Here's how the part is built. I have some questions about the finished solid (model axes, mm). A direction names the side the tool comes from. Round coordinates to 2 decimals unless told otherwise and drop trailing zeros. Order: outer loops, then holes, each group sorted by start corner. A loop starts at its lowest first (then second) coordinate and runs counter-clockwise, first axis right, second up. Notation, with made-up numbers: (55, -34) -> (90, -34) arc R18 ccw to (90, -30) -> close; hole circle Ø1 at (0.25, 68). An arc over 180 degrees is marked (long way). Use a Markdown table: item, result. Add a question column.
(1) I want a section at B-B, the plane z = -1. Please give me the cut outline in (x, y), then the cut area to 3 significant figures.
(2) I want a section at C-C, the plane x = 4. Give the number of separate pieces and of enclosed holes in the cut face, then the cut area to 3 significant figures.
(3) I want a section at A-A, the plane x = 0. Please give me the cut outline in (y, z), then the cut area to 3 significant figures.
(4) I'm going to push flat-ended pins straight in: P1, Ø10, axis at x = 2, z = -15.5, coming from the +Y side; P2, Ø4, axis at x = 12, y = 45.5, coming from the +Z side; P3, Ø5, axis at x = 4.5, y = 31, coming from the -Z side; P4, Ø10, axis at x = 2.5, z = -0.5, coming from the -Y side. Where does each tip first touch, or does it pass through?
(5) Thinking about a two-plate mould opening in Y: for faces 1 (the face through (-18.369, 29, 0)), 2 (the face through (-17.45, 36.35, -3.61)), 3 (the face through (0.861, 62.494, -16.123)), which applies, pulls with the +Y half, pulls with the -Y half, needs draft (parallel to the pull), parting line crosses it, or undercut?
(6) On a 3-axis mill with a long thin cutter (end or side, diameter ignored), from which of +Z, -Z, +X, -X, +Y, -Y can I reach the whole of each face in a straight line? I mean faces 4 (the face through (0, 28, 0)), 5 (the face through (1, 58, -21.7)), 6 (the face through (4.5, 58, -18)). Say none if no direction works.
(7) If I drill on probe 1 along X at (y, z) = (45, -7.5); probe 2 along Y at (x, z) = (0, -12.25); probe 3 along Y at (x, z) = (0, -9.25), over which ranges is the centre line in solid material (lowest first)?
(8) I want a section at D-D, the plane z = -8. Please give me the cut outline in (x, y), then the cut area to 3 significant figures.
Autodesk Inventor part; units mm, degrees
ref_plane "Work Plane2" through (0, 61, 0) normal (0, 1, 0) x (-1, 0, 0)
ref_plane "YZ Plane" through (0, 0, 0) normal (1, 0, 0) x (0, 1, 0)
ref_plane "XY Plane" through (0, 0, 0) normal (0, 0, 1) x (1, 0, 0)
sketch "Sketch1" plane through (0, 0, 0) normal (0, 0, 1) x (1, 0, 0)
  circle A0 centre (0, 0) radius 11
  line L0 (-9.5, 5.5453) -> (-9.5, -5.5453)
  line L1 (9.5, 5.5453) -> (9.5, -5.5453)
  circle A1 centre (0, 0) radius 32.5
  dimension "d0" = 22
  dimension "d1" = 19
  dimension "d2" = 65
extrude "Extrusion1" add sketch "Sketch1" along normal blind 3.3 contours A0 L1 | L0 A0 | A1
sketch "Sketch2" plane through (0, 0, 0) normal (1, 0, 0) x (0, 1, 0)
  line L0 (32.5, 0) -> (-32.5, 0)
  line L1 (32.5, 0) -> (55.5, -21.7)
  line L2 (55.5, -21.7) -> (62.5, -21.7)
  line L3 (62.5, -21.7) -> (62.5, -10.7)
  line L4 (32.5, 3.3) -> (-32.5, 3.3)
  line L5 (32.5, 3.3) -> (62.5, -10.7)
  line L6 (0, 0) -> (0, -19.375) construction
  line L7 (32.5, 3.3) -> (32.5, 0)
  dimension "d8" = 7
  dimension "d9" = 25
  dimension "d10" = 11
  dimension "d11" = 30
revolve "Revolution1" add sketch "Sketch2" angle 360 about axis through (0, 0, 0) along (0, 0, -1)
fillet "Fillet1" radius 10 1 edges at (0, -32.5, 3.3)
ref_plane "Work Plane2" through (0, 61, 0) normal (0, 1, 0) x (-1, 0, 0)
sketch "Sketch3" plane through (0, 61, 0) normal (0, 1, 0) x (-1, 0, 0)
  circle A0 centre (0, -16.2) radius 4.5
  line L0 (4.5, -16.2) -> (4.5, -20.7)
  line L1 (-4.5, -20.7) -> (-4.5, -16.2)
  line L2 (-62.5, -21.7) -> (62.5, -21.7)
  line L3 (62.5, -21.7) -> (62.5, -11.7) construction
  line L4 (62.5, -10.7) -> (62.5, -21.7)
  line L5 (-9.5, 0) -> (9.5, 0)
  line L6 (-4.5, -20.7) -> (4.5, -20.7)
  point P0 (0, 0)
  point P1 (0, 0)
  point P2 (0, -20.7)
  dimension "d14" = 9
  dimension "d22" = 1
extrude "Extrusion2" cut sketch "Sketch3" against normal blind 6
sketch "Sketch4" plane through (0, 0, 3.3) normal (0, 0, 1) x (1, 0, 0)
  circle A0 centre (0, 45) radius 9
  point P0 (0, 0)
  dimension "d25" = 45
  dimension "d26" = 18
extrude "Extrusion3" cut sketch "Sketch4" against normal through all
pattern_circular "Circular Pattern1" count 10 over 360 about axis through (0, 0, -6.7) along (0, 0, 1) of "Extrusion3"
sketch "Sketch5" plane through (0, 0, -21.7) normal (0, 0, -1) x (-1, 0, 0)
  line L0 (82.923, -74.4217) -> (-85.9985, -74.4217)
  line L1 (-85.9985, -74.4217) -> (-85.9985, 73.4258)
  line L2 (-85.9985, 73.4258) -> (82.923, 73.4258)
  line L3 (82.923, 73.4258) -> (82.923, -74.4217)
  line L4 (-19.4974, 63.9822) -> (18.3694, 63.9822)
  line L5 (18.3694, 63.9822) -> (18.3694, 24.2787)
  line L6 (18.3694, 24.2787) -> (-19.4974, 24.2787)
  line L7 (-19.4974, 24.2787) -> (-19.4974, 63.9822)
  point P0 (0, 0)
extrude "Extrusion4" cut sketch "Sketch5" against normal through all
properties part number "CVT_Ring"
Taken from the geometry:
| question | item | result |
|---|---|---|
| 1 | outline | (-18.37, 28.09) arc R33.56 cw to (19.5, 27.32) -> (19.5, 30.69) arc R9 cw to (17.56, 37.84) arc R41.71 ccw to (8.03, 40.93) arc R9 cw to (-8.03, 40.93) arc R41.71 ccw to (-17.56, 37.84) arc R9 cw to (-18.37, 32.44) -> close |
| 1 | area | 245 mm2 |
| 2 | separate pieces | 2 |
| 2 | enclosed holes | 1 |
| 2 | area | 127 mm2 |
| 3 | outline | (24.28, 0) -> (32.5, 0) -> (36, -3.3) -> (36, 1.67) -> (34.51, 2.36) arc R10 ccw to (30.28, 3.3) -> (24.28, 3.3) -> close; (54, -20.28) -> (55.5, -21.7) -> (62.5, -21.7) -> (62.5, -10.7) -> (54, -6.73) -> close; hole (55, -20.7) -> (61, -20.7) -> (61, -11.7) -> (55, -11.7) -> close |
| 3 | area | 96.5 mm2 |
| 4 | P1 | stops at y = 62.5 |
| 4 | P2 | stops at z = -2.56 |
| 4 | P3 | stops at z = -1.25 |
| 4 | P4 | stops at y = 24.28 |
| 5 | face 1 | needs draft |
| 5 | face 2 | undercut |
| 5 | face 3 | pulls with the +Y half |
| 6 | face 4 | -Z, -Y |
| 6 | face 5 | -Z, +X, -X, +Y, -Y |
| 6 | face 6 | none |
| 7 | probe 1 | x = -18.37 to -9, 9 to 19.5 |
| 7 | probe 2 | y = 54 to 55, 61 to 62.5 |
| 7 | probe 3 | y = 54 to 59.39 |
| 8 | outline | (-18.37, 40.37) arc R9 cw to (-17.47, 37.07) arc R40.98 cw to (-7.65, 40.26) arc R9 cw (long way) to (7.65, 40.26) arc R40.98 cw to (17.47, 37.07) arc R9 cw to (19.5, 42.12) -> (19.5, 53.26) arc R56.71 ccw to (-18.37, 53.66) -> close |
| 8 | area | 402 mm2 |
